Read the model definition and answer for the solid it produces. Units are mm, in the model's axes. Coordinates: 2 decimals unless noted, no trailing zeros. Write each loop counter-clockwise with the first axis right and the second up, starting at its lowest first coordinate (ties: lowest second). Pieces come first, ordered by that corner, then holes. Notation, with made-up numbers: (78, 67) - (112, 67) arc R29 ccw to (112, 92) - close; hole circle Ø7 at (70, -26). An arc over 180 degrees is marked (long way). Return JSON: item names as keys, results as strings.
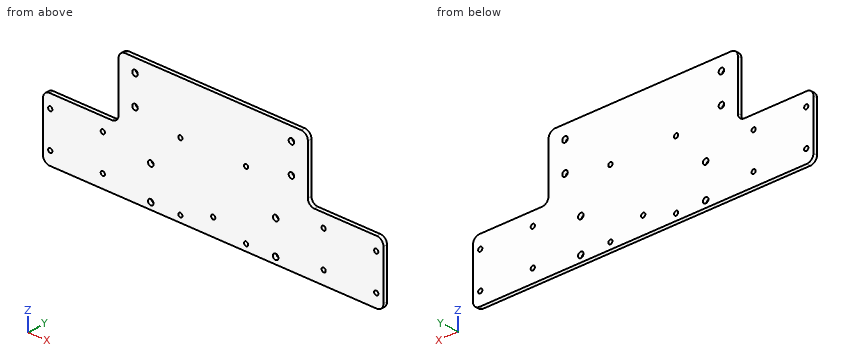
```python
from build123d import *

# Parameters (mm, degrees)
SKETCH_1_R       = 2.1
SKETCH_1_R_2     = 1.6
EXTRUDE_1_DEPTH  = 3
FILLET_START     = -1
FILLET_1_DEPTH   = 5
FILLET_1_2_DEPTH = 3


with BuildPart() as part:
    # Sketch 1 → Extrude 1 (new body)
    with BuildSketch(Plane.XZ):
        Polygon((-72, 0), (72, 0), (72, -47), (129.5, -47), (129.5, -94), (-129.5, -94), (-129.5, -47), (-72, -47), align=None)
        with Locations(Location((47.5, -89, 0), (0, 0, 90))):
            Circle(SKETCH_1_R, mode=Mode.SUBTRACT)
        with Locations(Location((-124, -84, 0), (0, 0, 90))):
            Circle(SKETCH_1_R_2, mode=Mode.SUBTRACT)
        with Locations(Location((-25, -89, 0), (0, 0, 270))):
            Circle(SKETCH_1_R_2, mode=Mode.SUBTRACT)
        with Locations(Location((-59.5, -32, 0), (0, 0, 90))):
            Circle(SKETCH_1_R, mode=Mode.SUBTRACT)
        with Locations(Location((-25, -39, 0), (0, 0, 270))):
            Circle(SKETCH_1_R_2, mode=Mode.SUBTRACT)
        with Locations(Location((84, -84, 0), (0, 0, 270))):
            Circle(SKETCH_1_R_2, mode=Mode.SUBTRACT)
        with Locations(Location((-59.5, -10, 0), (0, 0, 270))):
            Circle(SKETCH_1_R, mode=Mode.SUBTRACT)
        with Locations(Location((47.5, -64, 0), (0, 0, 90))):
            Circle(SKETCH_1_R, mode=Mode.SUBTRACT)
        with Locations(Location((-84, -57, 0), (0, 0, 270))):
            Circle(SKETCH_1_R_2, mode=Mode.SUBTRACT)
        with Locations(Location((-124, -57, 0), (0, 0, 270))):
            Circle(SKETCH_1_R_2, mode=Mode.SUBTRACT)
        with Locations(Location((-47.5, -64, 0), (0, 0, 270))):
            Circle(SKETCH_1_R, mode=Mode.SUBTRACT)
        with Locations(Location((-84, -84, 0), (0, 0, 90))):
            Circle(SKETCH_1_R_2, mode=Mode.SUBTRACT)
        with Locations(Location((124, -57, 0), (0, 0, 90))):
            Circle(SKETCH_1_R_2, mode=Mode.SUBTRACT)
        with Locations(Location((84, -57, 0), (0, 0, 90))):
            Circle(SKETCH_1_R_2, mode=Mode.SUBTRACT)
        with Locations(Location((59.5, -10, 0), (0, 0, 90))):
            Circle(SKETCH_1_R, mode=Mode.SUBTRACT)
        with Locations(Location((25, -39, 0), (0, 0, 90))):
            Circle(SKETCH_1_R_2, mode=Mode.SUBTRACT)
        with Locations(Location((59.5, -32, 0), (0, 0, 270))):
            Circle(SKETCH_1_R, mode=Mode.SUBTRACT)
        with Locations(Location((25, -89, 0), (0, 0, 90))):
            Circle(SKETCH_1_R_2, mode=Mode.SUBTRACT)
        with Locations(Location((124, -84, 0), (0, 0, 270))):
            Circle(SKETCH_1_R_2, mode=Mode.SUBTRACT)
        with Locations(Location((0, -81, 0), (0, 0, 270))):
            Circle(SKETCH_1_R_2, mode=Mode.SUBTRACT)
        with Locations(Location((-47.5, -89, 0), (0, 0, 270))):
            Circle(SKETCH_1_R, mode=Mode.SUBTRACT)
    extrude(amount=-EXTRUDE_1_DEPTH)

    # Fillet 1: read off the stored shape, not the designer's step
    # Fillet 1 outline → Fillet 1 (cut)
    with BuildSketch(Plane(origin=(0, 0, 0), x_dir=(1, 0, 0), z_dir=(0, 1, 0)).offset(FILLET_START)):
        with BuildLine():
            Line((72, 0), (72, 5))
            add(Edge.make_bspline(
                [(72, 5), (72, 0), (67, 0)],
                knots=[0, 0, 0, 1, 1, 1], degree=2, weights=[1, 0.707106781, 1]))
            Line((67, 0), (72, 0))
        make_face()
        with BuildLine():
            Line((-72, 0), (-67, 0))
            add(Edge.make_bspline(
                [(-67, 0), (-72, 0), (-72, 5)],
                knots=[0, 0, 0, 1, 1, 1], degree=2, weights=[1, 0.707106781, 1]))
            Line((-72, 5), (-72, 0))
        make_face()
        with BuildLine():
            add(Edge.make_bspline(
                [(129.5, 52), (129.5, 47), (124.5, 47)],
                knots=[0, 0, 0, 1, 1, 1], degree=2, weights=[1, 0.707106781, 1]))
            Line((124.5, 47), (129.5, 47))
            Line((129.5, 47), (129.5, 52))
        make_face()
        with BuildLine():
            add(Edge.make_bspline(
                [(124.5, 94), (129.5, 94), (129.5, 89)],
                knots=[0, 0, 0, 1, 1, 1], degree=2, weights=[1, 0.707106781, 1]))
            Line((129.5, 89), (129.5, 94))
            Line((129.5, 94), (124.5, 94))
        make_face()
        with BuildLine():
            Line((-129.5, 47), (-124.5, 47))
            add(Edge.make_bspline(
                [(-124.5, 47), (-129.5, 47), (-129.5, 52)],
                knots=[0, 0, 0, 1, 1, 1], degree=2, weights=[1, 0.707106781, 1]))
            Line((-129.5, 52), (-129.5, 47))
        make_face()
        with BuildLine():
            add(Edge.make_bspline(
                [(-129.5, 89), (-129.5, 94), (-124.5, 94)],
                knots=[0, 0, 0, 1, 1, 1], degree=2, weights=[1, 0.707106781, 1]))
            Line((-124.5, 94), (-129.5, 94))
            Line((-129.5, 94), (-129.5, 89))
        make_face()
    extrude(amount=FILLET_1_DEPTH, mode=Mode.SUBTRACT)

    # Fillet 1 2 outline → Fillet 1 2 (add)
    with BuildSketch(Plane(origin=(0, 0, 0), x_dir=(1, 0, 0), z_dir=(0, 1, 0))):
        with BuildLine():
            Line((72, 47), (72, 42))
            add(Edge.make_bspline(
                [(77, 47), (72, 47), (72, 42)],
                knots=[0, 0, 0, 1, 1, 1], degree=2, weights=[1, 0.707106781, 1]))
            Line((77, 47), (72, 47))
        make_face()
        with BuildLine():
            add(Edge.make_bspline(
                [(-72, 42), (-72, 47), (-77, 47)],
                knots=[0, 0, 0, 1, 1, 1], degree=2, weights=[1, 0.707106781, 1]))
            Line((-72, 42), (-72, 47))
            Line((-72, 47), (-77, 47))
        make_face()
    extrude(amount=FILLET_1_2_DEPTH)


solid = part.part
```
(1) Flat-ended cylindrical pins translate along their axes: P1, Ø1.5, axis at x = 41, y = 1, coming from the +Z side; P2, Ø1.5, axis at x = 96.5, y = 1.5, coming from the +Z side; P3, Ø1, axis at y = 2, z = -17, coming from the -X side. Find the tip coordinate at first contact, or state that the pin passes through.
Answer:
{"P1": "z = 0", "P2": "z = -47", "P3": "x = -72"}
(2) A cutting plane is placed at C-C (x = 91). Determine the outline of the cut face in (y, z), and give its area (3 significant figures).
Answer:
{"outline": "(0, -94) - (3, -94) - (3, -47) - (0, -47) - close", "area": "141 mm²"}
(3) A cutting plane is placed at A-A (z = -18). Determine the outline of the cut face in (x, y), and give its area (3 significant figures).
Answer:
{"outline": "(-72, 0) - (72, 0) - (72, 3) - (-72, 3) - close", "area": "432 mm²"}
(4) Straight lines are drawn through the part: line 1 (X direction, y = 1.95, z = -39); line 2 (X direction, y = 2.35, z = -84); line 3 (Z direction, x = 47.5, y = 0.6). For each, find the intervals that lie inside material, in ascending order. Write a range as from..to.
Answer:
{"line 1": "-72..-26.6, -23.4..23.4, 26.6..72", "line 2": "-129.5..-125.6, -122.4..-85.6, -82.4..82.4, 85.6..122.4, 125.6..129.5", "line 3": "-94..-91.1, -86.9..-66.1, -61.9..0"}
(5) A cutting plane is placed at B-B (y = 2.2). State how many separate pieces and enclosed holes the cut face has, and give its area (3 significant figures).
Answer:
{"separate pieces": "1", "enclosed holes": "21", "area": "18,700 mm²"}
